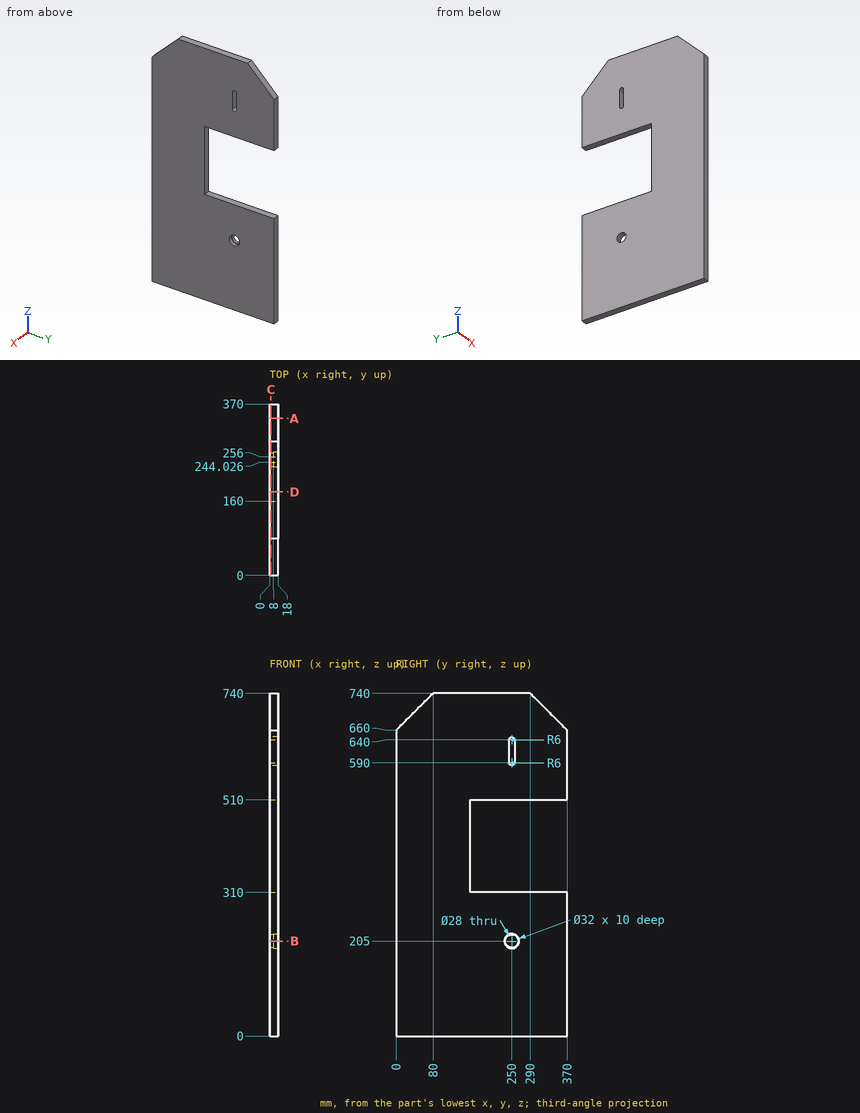
Print and shaded views of the part. All mm, measured from the part's lowest x, y and z. Coordinates: 2 decimals unless noted, no trailing zeros. Order: outer loops, then holes, each group sorted by start corner. A loop starts at its lowest first (then second) coordinate and runs counter-clockwise, first axis right, second up. Notation, with made-up numbers: (67.25, -30) - (122.25, -30) arc R7 ccw to (122.25, -24) - close; hole circle Ø6 at (-9, -34). An arc over 180 degrees is marked (long way). Put each result on its own line as item: value.
1. Drop flat-ended pins along their axis: P1, Ø5, axis at y = 315, z = 268.5, coming from the -X side; P2, Ø5, axis at x = 14, y = 330, coming from the +Z side. Give the stop position or say it passes through.
Answer sheet:
P1: stops at x = 0
P2: stops at z = 702.5
2. Saw through at B-B (z = 205). Write the cut outline in (x, y).
Answer sheet:
outline: (0, 0) - (18, 0) - (18, 234) - (8, 234) - (8, 236) - (0, 236) - close; (0, 264) - (8, 264) - (8, 266) - (18, 266) - (18, 370) - (0, 370) - close
3. Saw through at C-C (x = 2.75). Write the cut outline in (y, z).
Answer sheet:
outline: (0, 0) - (370, 0) - (370, 310) - (160, 310) - (160, 510) - (370, 510) - (370, 660) - (290, 740) - (80, 740) - (0, 660) - close; hole circle Ø28 at (250, 205); hole (244.03, 589.44) arc R6 ccw to (256, 590) - (256, 640) arc R6 ccw to (244.03, 640.56) arc R6 ccw to (244.03, 639.44) - (244.03, 590.56) arc R6 ccw to start
4. Saw through at D-D (y = 180). Write the cut outline in (x, z), and give its area (3 significant figures).
Answer sheet:
outline: (0, 0) - (18, 0) - (18, 310) - (0, 310) - close; (0, 510) - (18, 510) - (18, 740) - (0, 740) - close
area: 9,720 mm^2
5. Probe line 1 along Z through (x, y) = (6.25, 250); line 2 along Z through (x, y) = (6.5, 168); line 3 along Z through (x, y) = (12.75, 330). List the from-to ranges inside material, lowest first. Write a range as [from, to].
Answer sheet:
line 1: z = [0, 191], [219, 310], [510, 584], [646, 740]
line 2: z = [0, 310], [510, 740]
line 3: z = [0, 310], [510, 700]
6. Saw through at A-A (y = 339). Write the cut outline in (x, z), and give its area (3 significant figures).
Answer sheet:
outline: (0, 0) - (18, 0) - (18, 310) - (0, 310) - close; (0, 510) - (18, 510) - (18, 691) - (0, 691) - close
area: 8,840 mm^2
